```python
from build123d import *

# Parameters (mm, degrees)
SKETCH2_R           = 58
BOSS_EXTRUDE1_DEPTH = 41.5
SKETCH3_R           = 48
CUT_EXTRUDE1_DEPTH  = 34
SKETCH4_R           = 3.175
CUT_EXTRUDE2_DEPTH  = 89.791891522
CUT_EXTRUDE3_DEPTH  = 92.925241365
SKETCH6_W           = 11
SKETCH6_H           = 25.4
CUT_EXTRUDE4_DEPTH  = 25
CIRPATTERN1_COUNT   = 9
SKETCH7_R           = 2.2
CUT_EXTRUDE5_DEPTH  = 86.500040351
CIRPATTERN2_COUNT   = 9
SKETCH8_R           = 11
CUT_EXTRUDE6_DEPTH  = 92.925241365


with BuildPart() as part:
    # Sketch2 → Boss-Extrude1 (new body)
    with BuildSketch(Plane(origin=(0, 0, 0), x_dir=(1, 0, 0), z_dir=(0, 1, 0))):
        with Locations(Location((0, 0, 0), (0, 0, 270))):
            Circle(SKETCH2_R)
    extrude(amount=BOSS_EXTRUDE1_DEPTH)

    # Sketch3 → Cut-Extrude1 (cut)
    with BuildSketch(Plane(origin=(0, 41.5, 0), x_dir=(1, 0, 0), z_dir=(0, 1, 0))):
        with Locations(Location((0, 0, 0), (0, 0, 270))):
            Circle(SKETCH3_R)
    extrude(amount=-CUT_EXTRUDE1_DEPTH, mode=Mode.SUBTRACT)

    # Sketch4 → Cut-Extrude2 (cut, through all)
    with BuildSketch(Plane(origin=(0, 7.5, 0), x_dir=(1, 0, 0), z_dir=(0, 1, 0))):
        with Locations(Location((0, 0, 0), (0, 0, 270))):
            Circle(SKETCH4_R)
    extrude(amount=-CUT_EXTRUDE2_DEPTH, mode=Mode.SUBTRACT)

    # Sketch5 → Cut-Extrude3 (cut, through all)
    with BuildSketch(Plane.XZ):
        with BuildLine():
            Line((12.851665748, -10.023238623), (19.92273356, -17.094306435))
            ThreePointArc((19.92273356, -17.094306435), (19.92273356, -19.92273356), (17.094306435, -19.92273356))
            Line((17.094306435, -19.92273356), (10.023238623, -12.851665748))
            ThreePointArc((10.023238623, -12.851665748), (10.023238623, -10.023238623), (12.851665748, -10.023238623))
        make_face()
        with BuildLine():
            Line((10.023238623, 12.851665748), (17.094306435, 19.92273356))
            ThreePointArc((17.094306435, 19.92273356), (19.92273356, 19.92273356), (19.92273356, 17.094306435))
            Line((19.92273356, 17.094306435), (12.851665748, 10.023238623))
            ThreePointArc((12.851665748, 10.023238623), (10.023238623, 10.023238623), (10.023238623, 12.851665748))
        make_face()
        with BuildLine():
            Line((-10.023238623, 12.851665748), (-17.094306435, 19.92273356))
            ThreePointArc((-17.094306435, 19.92273356), (-19.92273356, 19.92273356), (-19.92273356, 17.094306435))
            Line((-19.92273356, 17.094306435), (-12.851665748, 10.023238623))
            ThreePointArc((-12.851665748, 10.023238623), (-10.023238623, 10.023238623), (-10.023238623, 12.851665748))
        make_face()
        with BuildLine():
            Line((-12.851665748, -10.023238623), (-19.92273356, -17.094306435))
            ThreePointArc((-19.92273356, -17.094306435), (-19.92273356, -19.92273356), (-17.094306435, -19.92273356))
            Line((-17.094306435, -19.92273356), (-10.023238623, -12.851665748))
            ThreePointArc((-10.023238623, -12.851665748), (-10.023238623, -10.023238623), (-12.851665748, -10.023238623))
        make_face()
    extrude(amount=-CUT_EXTRUDE3_DEPTH, mode=Mode.SUBTRACT)

    # Sketch6 → Cut-Extrude4 (cut)
    with BuildSketch(Plane.XY.offset(58.000000078)):
        with Locations((-2.325, 11.43)):
            Rectangle(SKETCH6_W, SKETCH6_H)
    cut_extrude4 = extrude(amount=-CUT_EXTRUDE4_DEPTH, mode=Mode.SUBTRACT)

    # CirPattern1: Cut-Extrude4 ×9 about axis
    cirpattern1_axis = Axis((0, 0, 0), (0, 1, 0))
    for i in range(1, CIRPATTERN1_COUNT):
        add(cut_extrude4.rotate(cirpattern1_axis, i * 360 / CIRPATTERN1_COUNT), mode=Mode.SUBTRACT)

    # Sketch7 → Cut-Extrude5 (cut, through all)
    with BuildSketch(Plane.XZ.offset(-24.13)):
        with Locations(Location((-2.335541758, 52.90395562, 0), (0, 0, 270))):
            Circle(SKETCH7_R)
    cut_extrude5 = extrude(amount=-CUT_EXTRUDE5_DEPTH, mode=Mode.SUBTRACT)

    # CirPattern2: Cut-Extrude5 ×9 about axis
    cirpattern2_axis = Axis((0, 0, 0), (0, 1, 0))
    for i in range(1, CIRPATTERN2_COUNT):
        add(cut_extrude5.rotate(cirpattern2_axis, i * 360 / CIRPATTERN2_COUNT), mode=Mode.SUBTRACT)

    # Sketch8 → Cut-Extrude6 (cut, through all)
    with BuildSketch(Plane.XZ):
        with Locations(Location((0, 0, 0), (0, 0, 270))):
            Circle(SKETCH8_R)
    extrude(amount=-CUT_EXTRUDE6_DEPTH, mode=Mode.SUBTRACT)


solid = part.part
```
Part model, mm, in its own coordinate system. A direction names the side the tool comes from. Give positions to 0.01 mm unless a question says otherwise; leave off trailing zeros. Write each loop counter-clockwise with the first axis right and the second up, starting at its lowest first coordinate (ties: lowest second). Pieces come first, ordered by that corner, then holes. Notation, with made-up numbers: M 47,-31.75 L 87,-31.75 A26 ccw 87,0.25 Z; hole C 42.5,-34.5 d5. An arc over 180 degrees is marked long. Use CSV: the item, a comma, the result in double quotes.
Item 1: Drill centre lines: probe 1 along X at (y, z) = (39, -1); probe 2 along X at (y, z) = (27, -25); probe 3 along X at (y, z) = (32, 39). Where is each one in solid material? Low to high.
Taken from the geometry:
probe 1,"x = -57.99 to -47.99, 47.99 to 57.99"
probe 2,"x = -52.34 to -40.98, 40.98 to 44.86, 49.11 to 52.34"
probe 3,"x = -42.93 to -37.99, -33.6 to -27.98, 27.98 to 42.93"
Item 2: Slice it at B-B on y = 30. State how many separate pieces and enclosed holes the cut face has, plus the area to 3 significant figures.
Taken from the geometry:
separate pieces,"1"
enclosed holes,"10"
area,"3,190 mm²"
Item 3: Which spindle directions (+Z, -Z, +X, -X, +Y, -Y) get a long thin tool onto all of the face, cutting with end or side? Do faces 1 (the face through (-13.51, 3.7, 16.34)), 2 (the face through (24.94, 9.215, 41.896)), 3 (the face through (11.3, 7.5, -0.7)). Say none if no direction does.
Taken from the geometry:
face 1,"+Y, -Y"
face 2,"-Y"
face 3,"+Y"
Item 4: Pull direction Z, two halves, no side cores. Call faces 4 (the face through (-22.21, 20.46, 53.58)), 5 (the face through (-47.11, 9.21, 11.53)), 6 (the face through (-2, 4, 33)), 7 (the face through (-10.055, 3.698, 9.992)): +Z half, -Z half, draft (parallel to the pull), parting line (faces both ways), or undercut.
Taken from the geometry:
face 4,"parting line"
face 5,"undercut"
face 6,"+Z half"
face 7,"undercut"
Item 5: Slice it at A-A on x = 38. Write the cut outline in (y, z).
Taken from the geometry:
outline,"M 0,-43.82 L 41.5,-43.82 L 41.5,-29.33 L 7.5,-29.33 L 7.5,-25.61 L 0,-25.61 Z; M 0,-12.9 L 7.5,-12.9 L 7.5,3.48 L 0,3.48 Z; M 0,14.65 L 7.5,14.65 L 7.5,29.33 L 41.5,29.33 L 41.5,43.82 L 24.13,43.82 L 24.13,40.35 L 0,40.35 Z"
Item 6: Pin check, flat tips, straight feed: P1, Ø12, axis at x = -45.5, y = 9.5, coming from the -Z side; P2, Ø3, axis at x = 9.5, y = 21.5, coming from the +Z side; P3, Ø7, axis at y = 15.5, z = 46, coming from the +X side. Stop position of each tip, or through.
Taken from the geometry:
P1,"stops at z = -42.47"
P2,"stops at z = 57.45"
P3,"stops at x = 30.95"
